Work out the finished part from the listing and answer in its coordinate system (mm). Face numbers are marked on the shaded views. A direction names the side the tool comes from. Coordinates: 2 decimals unless noted, no trailing zeros. Loops run counter-clockwise (first coordinate to the right, second up) from the corner with the lowest first, then second, coordinate; pieces in that order, holes last. Notation, with made-up numbers: (-13.75, 21.25) - (18.25, 21.25) arc R34 ccw to (18.25, 54.25) - close; hole circle Ø2 at (42.5, 82). An arc over 180 degrees is marked (long way). Write each question's results on one line, items separated by ' | '. Start each with the question number.
1. Find the intervals of material crossed by line 1 along X through (y, z) = (2.8, 8.5); line 2 along X through (y, z) = (4.5, 11); line 3 along Z through (x, y) = (10, 2.65), in increasing order. Write a range as [from, to].
2. Which of the six approach directions +Z, -Z, +X, -X, +Y, -Y give full straight-line access (tool end or side, diameter ignored) to the marked faces 1, 2 and 3?
3. Each of these flat-tipped pins is pushed along its axis until it touches: P1, Ø3, axis at x = -7, y = 7, coming from the -Z side; P2, Ø5, axis at x = 4, z = 30.5, coming from the -Y side; P3, Ø1.9, axis at x = -5.5, z = 8.5, coming from the +Y side. Where does it stop, or does it pass through?
4. Determine the mould class of the marked faces 4, 5 and 6 for opening direction X: released by +X, released by -X, zero draft, split by the parting line, or undercut.
5. A cutting plane is placed at D-D on z = 11.75. Determine the outline of the cut face in (x, y).
6. A cutting plane is placed at B-B on x = -19.5. Determine the outline of the cut face in (y, z).
7. A cutting plane is placed at C-C on y = 6.75. Determine the outline of the cut face in (x, z), then the cut area to 3 significant figures.
8. A cutting plane is placed at A-A on z = 8.5. Determine the outline of the cut face in (x, y), then the cut area to 3 significant figures.
from build123d import *

# Parameters (mm, degrees)
SKETCH_1_W          = 54.664318292
SKETCH_1_H          = 5
SKETCH_1_R          = 1.5
EXTRUDE_1_DEPTH     = 5
SKETCH_2_W          = 59.460193076
SKETCH_2_H          = 2.500348526
EXTRUDE_2_DEPTH     = 23
SKETCH_5_R          = 16.5
CUT_EXTRUDE_1_DEPTH = 15
EXTRUDE_START       = 5
EXTRUDE_3_DEPTH     = 5
CHAMFER_1_SIZE      = 5
FILLET_6_R          = 10
FILLET_7_R          = 5
FILLET_8_R          = 3


with BuildPart() as part:
    # 草图1 → 凸台-拉伸1 (new body)
    with BuildSketch(Plane(origin=(0, 0, 0), x_dir=(1, 0, 0), z_dir=(0, 1, 0))):
        with Locations((1.075531559, -8.61)):
            Rectangle(SKETCH_1_W, SKETCH_1_H)
        with Locations(Location((-10, -8.5, 0), (0, 0, 270))):
            Circle(SKETCH_1_R, mode=Mode.SUBTRACT)
        with Locations(Location((10, -8.5, 0), (0, 0, 90))):
            Circle(SKETCH_1_R, mode=Mode.SUBTRACT)
    extrude(amount=EXTRUDE_1_DEPTH)

    # 草图2 → 凸台-拉伸2 (add)
    with BuildSketch(Plane.XY.offset(11.11)):
        with Locations((0, 2.5)):
            Rectangle(SKETCH_2_W, SKETCH_2_H)
    extrude(amount=EXTRUDE_2_DEPTH)

    # 草图5 → 切除-拉伸1 (cut)
    with BuildSketch(Plane(origin=(0, 3.750174263, 0), x_dir=(1, 0, 0), z_dir=(0, 1, 0))):
        with Locations((-0.32, -44.994124541)):
            Circle(SKETCH_5_R)
    extrude(amount=-CUT_EXTRUDE_1_DEPTH, mode=Mode.SUBTRACT)

    # 草图7 → 凸台-拉伸3 (add)
    with BuildSketch(Plane(origin=(0, 3.750174263, 0), x_dir=(1, 0, 0), z_dir=(0, 1, 0)).offset(EXTRUDE_START)):
        with BuildLine():
            Line((-29.730096538, -34.11), (-12.721041608, -34.11))
            ThreePointArc((-12.721041608, -34.11), (-0.32, -28.494124541), (12.081041608, -34.11))
            Line((12.081041608, -34.11), (29.730096538, -34.11))
            Line((29.730096538, -34.11), (29.730096538, -11.11))
            Line((29.730096538, -11.11), (28.407690705, -11.11))
            Line((28.407690705, -11.11), (-26.256627587, -11.11))
            Line((-26.256627587, -11.11), (-29.730096538, -11.11))
            Line((-29.730096538, -11.11), (-29.730096538, -34.11))
        make_face()
    extrude(amount=-EXTRUDE_3_DEPTH)

    # 倒角1
    # the kernel refuses this chamfer: 5 mm, written as the material it takes off along each edge
    with BuildSketch(Plane(origin=(-42.588511478, 8.750174263, 11.11), x_dir=(0, -0.9996219169112968, -0.027495876610586317), z_dir=(1, 0, 0))) as chamfer_1_piece_1_section:
        Polygon((CHAMFER_1_SIZE * 0.999621916911, -CHAMFER_1_SIZE * 0.0274958766106), (-CHAMFER_1_SIZE * 0.0274958766106, -CHAMFER_1_SIZE * 0.999621916911), (0, 0), align=None)
    chamfer_1_piece_1 = extrude(amount=85.177022955, mode=Mode.PRIVATE)
    chamfer_1_piece_1 = split(chamfer_1_piece_1, bisect_by=Plane(origin=(-34.422569532, 5, 11.399404242), z_dir=(0, -1, 0)), keep=Keep.TOP, mode=Mode.PRIVATE)
    chamfer_1_piece_1 = split(chamfer_1_piece_1, bisect_by=Plane(origin=(-26.256627587, 4.506210637, 11.399404242), z_dir=(-1, 0, 0)), keep=Keep.TOP, mode=Mode.PRIVATE)
    add(chamfer_1_piece_1, mode=Mode.SUBTRACT)
    with BuildSketch(Plane(origin=(-42.588511478, 8.750174263, 11.11), x_dir=(0, -0.9996219169112968, -0.027495876610586317), z_dir=(1, 0, 0))) as chamfer_1_piece_2_section:
        Polygon((CHAMFER_1_SIZE * 0.999621916911, -CHAMFER_1_SIZE * 0.0274958766106), (-CHAMFER_1_SIZE * 0.0274958766106, -CHAMFER_1_SIZE * 0.999621916911), (0, 0), align=None)
    chamfer_1_piece_2 = extrude(amount=85.177022955, mode=Mode.PRIVATE)
    chamfer_1_piece_2 = split(chamfer_1_piece_2, bisect_by=Plane(origin=(-34.422569532, 5, 12.869772417), z_dir=(0, 1, 0)), keep=Keep.TOP, mode=Mode.PRIVATE)
    chamfer_1_piece_2 = split(chamfer_1_piece_2, bisect_by=Plane(origin=(-26.256627587, 7.312697929, 12.869772417), z_dir=(-1, 0, 0)), keep=Keep.TOP, mode=Mode.PRIVATE)
    add(chamfer_1_piece_2, mode=Mode.SUBTRACT)
    with BuildSketch(Plane(origin=(-42.588511478, 8.750174263, 11.11), x_dir=(0, -0.9996219169112968, -0.027495876610586317), z_dir=(1, 0, 0))) as chamfer_1_piece_3_section:
        Polygon((CHAMFER_1_SIZE * 0.999621916911, -CHAMFER_1_SIZE * 0.0274958766106), (-CHAMFER_1_SIZE * 0.0274958766106, -CHAMFER_1_SIZE * 0.999621916911), (0, 0), align=None)
    chamfer_1_piece_3 = extrude(amount=85.177022955, mode=Mode.PRIVATE)
    chamfer_1_piece_3 = split(chamfer_1_piece_3, bisect_by=Plane(origin=(1.075531559, 5, 12.869772417), z_dir=(0, 1, 0)), keep=Keep.TOP, mode=Mode.PRIVATE)
    chamfer_1_piece_3 = split(chamfer_1_piece_3, bisect_by=Plane(origin=(28.407690705, 7.312697929, 12.869772417), z_dir=(-1, 0, 0)), keep=Keep.TOP, mode=Mode.PRIVATE)
    chamfer_1_piece_3 = split(chamfer_1_piece_3, bisect_by=Plane(origin=(-26.256627587, 7.312697929, 12.869772417), z_dir=(1, 0, 0)), keep=Keep.TOP, mode=Mode.PRIVATE)
    add(chamfer_1_piece_3, mode=Mode.SUBTRACT)
    with BuildSketch(Plane(origin=(-42.588511478, 8.750174263, 11.11), x_dir=(0, -0.9996219169112968, -0.027495876610586317), z_dir=(1, 0, 0))) as chamfer_1_piece_4_section:
        Polygon((CHAMFER_1_SIZE * 0.999621916911, -CHAMFER_1_SIZE * 0.0274958766106), (-CHAMFER_1_SIZE * 0.0274958766106, -CHAMFER_1_SIZE * 0.999621916911), (0, 0), align=None)
    chamfer_1_piece_4 = extrude(amount=85.177022955, mode=Mode.PRIVATE)
    chamfer_1_piece_4 = split(chamfer_1_piece_4, bisect_by=Plane(origin=(35.498101091, 5, 11.399404242), z_dir=(0, -1, 0)), keep=Keep.TOP, mode=Mode.PRIVATE)
    chamfer_1_piece_4 = split(chamfer_1_piece_4, bisect_by=Plane(origin=(28.407690705, 4.506210637, 11.399404242), z_dir=(1, 0, 0)), keep=Keep.TOP, mode=Mode.PRIVATE)
    add(chamfer_1_piece_4, mode=Mode.SUBTRACT)
    with BuildSketch(Plane(origin=(-42.588511478, 8.750174263, 11.11), x_dir=(0, -0.9996219169112968, -0.027495876610586317), z_dir=(1, 0, 0))) as chamfer_1_piece_5_section:
        Polygon((CHAMFER_1_SIZE * 0.999621916911, -CHAMFER_1_SIZE * 0.0274958766106), (-CHAMFER_1_SIZE * 0.0274958766106, -CHAMFER_1_SIZE * 0.999621916911), (0, 0), align=None)
    chamfer_1_piece_5 = extrude(amount=85.177022955, mode=Mode.PRIVATE)
    chamfer_1_piece_5 = split(chamfer_1_piece_5, bisect_by=Plane(origin=(35.498101091, 5, 12.869772417), z_dir=(0, 1, 0)), keep=Keep.TOP, mode=Mode.PRIVATE)
    chamfer_1_piece_5 = split(chamfer_1_piece_5, bisect_by=Plane(origin=(28.407690705, 7.312697929, 12.869772417), z_dir=(1, 0, 0)), keep=Keep.TOP, mode=Mode.PRIVATE)
    add(chamfer_1_piece_5, mode=Mode.SUBTRACT)

    # 圆角6
    # the kernel refuses this fillet: 10 mm, written as the material it adds along each edge
    with BuildSketch(Plane(origin=(28.407690705, 1.249825737, 11.11), x_dir=(0, 0, 1), z_dir=(-1, 0, 0))) as fillet_6_piece_1:
        with BuildLine():
            CenterArc((4.840914208, -10), FILLET_6_R, 90, 28.952961909)
            Line((0, -1.249825737), (0, 0))
            Line((0, 0), (4.840914208, 0))
        make_face()
    extrude(amount=54.664318292)

    # 圆角7
    fillet_7_edges = [part.edges().sort_by_distance(p)[0] for p in [
        (-12.721041608, 5, 34.11),
        (12.081041608, 5, 34.11),
    ]]
    fillet(fillet_7_edges, radius=FILLET_7_R)

    # 圆角8
    fillet_8_edges = [part.edges().sort_by_distance(p)[0] for p in [
        (-0.32, 1.249825737, 28.494124541),
        (21.949780623, 1.249825737, 34.11),
        (-13.002521469, 1.249825737, 33.772076375),
        (12.362521469, 1.249825737, 33.772076375),
        (-22.269780623, 1.249825737, 34.11),
    ]]
    fillet(fillet_8_edges, radius=FILLET_8_R)


solid = part.part
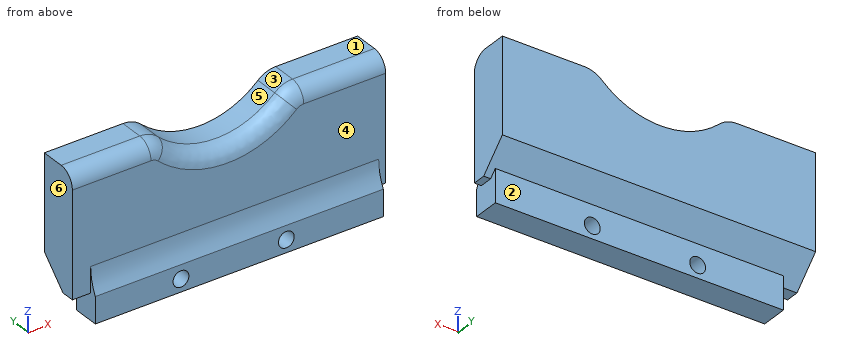
Values:
1) line 1: [-26.26, -11.5], [-8.5, 8.5], [11.5, 28.41] | line 2: [-26.26, 28.41] | line 3: [6.11, 7], [10, 31.53]
2) face 1: +Z, +X, -X, +Y, -Y | face 2: -Z, +X, -X, +Y | face 3: +Z, +Y, -Y
3) P1: z = 12.86 | P2: y = 1.91 | P3: y = 5
4) face 4: zero draft | face 5: undercut | face 6: released by -X
5) outline: (-29.73, 1.25) - (-26.26, 1.25) - (-26.26, 0.32) - (28.41, 0.32) - (28.41, 1.25) - (29.73, 1.25) - (29.73, 4.39) - (28.41, 4.39) - (28.41, 5) - (-26.26, 5) - (-26.26, 4.39) - (-29.73, 4.39) - close
6) outline: (0, 6.11) - (5, 6.11) - (5, 12.36) - (8.75, 16.11) - (8.75, 34.11) - (4.25, 34.11) arc R3 ccw to (1.25, 31.11) - (1.25, 15.95) arc R10 cw to (0, 11.11) - close
7) outline: (-29.73, 14.11) - (29.73, 14.11) - (29.73, 34.11) - (14.17, 34.11) arc R5 ccw to (10.8, 32.8) arc R16.5 cw to (-11.44, 32.8) arc R5 ccw to (-14.81, 34.11) - (-29.73, 34.11) - close | area: 1,090 mm^2
8) outline: (-26.26, 0) - (-11.5, 0) - (-11.5, 5) - (-26.26, 5) - close; (-8.5, 0) - (8.5, 0) - (8.5, 5) - (-8.5, 5) - close; (11.5, 0) - (28.41, 0) - (28.41, 5) - (11.5, 5) - close | area: 243 mm^2
